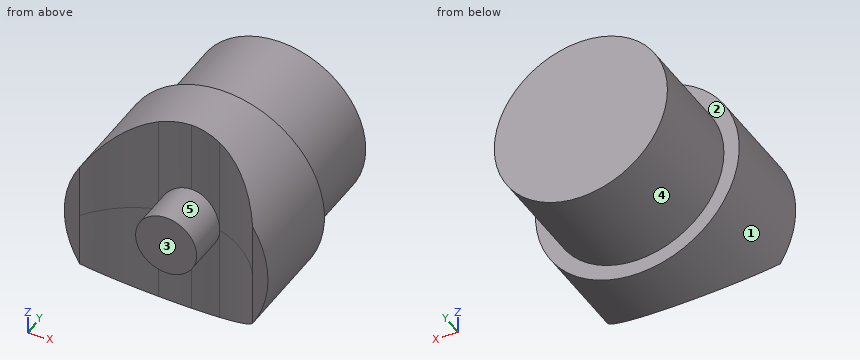
```python
from build123d import *

# Parameters (mm, degrees)
F0_W          = 1.5
F0_H          = 10
F0_W_2        = 8.5
F2_DEPTH      = 25
F2_DEPTH_BACK = 25


with BuildPart() as f1:
    # F0 (on Top) → F1 (revolve)
    with BuildSketch(Plane.XY):
        with BuildLine():
            Line((-10, 10), (-18.5, 10))
            Line((-18.5, 10), (-18.5, 0))
            ThreePointArc((-18.5, 0), (-16.099974277, 2.509062325), (-13, 4.0729282733))
            Line((-13, 4.0729282733), (-13, 4.5217803813))
            Line((-13, 4.5217803813), (-10, 4.5217803813))
            Line((-10, 4.5217803813), (-10, 10))
        make_face()
        with Locations((-19.25, 5)):
            Rectangle(F0_W, F0_H)
        with Locations((-14.25, 15)):
            Rectangle(F0_W_2, F0_H)
        with BuildLine():
            ThreePointArc((-13, 4.0729282733), (-11.516696098, 4.4089463041), (-10, 4.5217803813))
            Line((-10, 4.5217803813), (-13, 4.5217803813))
            Line((-13, 4.5217803813), (-13, 4.0729282733))
        make_face()
        with BuildLine():
            Line((-10, 0), (-10, 4.5217803813))
            ThreePointArc((-10, 4.5217803813), (-11.516696098, 4.4089463041), (-13, 4.0729282733))
            Line((-13, 4.0729282733), (-13, 0))
            Line((-13, 0), (-10, 0))
        make_face()
        with BuildLine():
            ThreePointArc((-13, 4.0729282733), (-16.099974277, 2.509062325), (-18.5, 0))
            Line((-18.5, 0), (-13, 0))
            Line((-13, 0), (-13, 4.0729282733))
        make_face()
    revolve(axis=Axis((-10, 10, 0), (0, -1, 0)))

    # F0 (on Top) → F2 (cut, two sides)
    with BuildSketch(Plane.XY) as f2_sk:
        with BuildLine():
            ThreePointArc((-13, 4.0729282733), (-16.099974277, 2.509062325), (-18.5, 0))
            Line((-18.5, 0), (-13, 0))
            Line((-13, 0), (-13, 4.0729282733))
        make_face()
        with BuildLine():
            Line((-7, 0), (-1.5, 0))
            ThreePointArc((-1.5, 0), (-3.900025723, 2.509062325), (-7, 4.0729282733))
            Line((-7, 4.0729282733), (-7, 0))
        make_face()
        with BuildLine():
            Line((-10, 0), (-10, 4.5217803813))
            ThreePointArc((-10, 4.5217803813), (-11.516696098, 4.4089463041), (-13, 4.0729282733))
            Line((-13, 4.0729282733), (-13, 0))
            Line((-13, 0), (-10, 0))
        make_face()
        with BuildLine():
            ThreePointArc((-7, 4.0729282733), (-8.483303902, 4.4089463041), (-10, 4.5217803813))
            Line((-10, 4.5217803813), (-10, 0))
            Line((-10, 0), (-7, 0))
            Line((-7, 0), (-7, 4.0729282733))
        make_face()
    extrude(amount=F2_DEPTH, mode=Mode.SUBTRACT)
    extrude(f2_sk.sketch, amount=-F2_DEPTH_BACK, mode=Mode.SUBTRACT)

    # F0 (on Top) → F3 (revolve)
    with BuildSketch(Plane.XY):
        with BuildLine():
            Line((-10, 0), (-10, 4.5217803813))
            ThreePointArc((-10, 4.5217803813), (-11.516696098, 4.4089463041), (-13, 4.0729282733))
            Line((-13, 4.0729282733), (-13, 0))
            Line((-13, 0), (-10, 0))
        make_face()
        with BuildLine():
            ThreePointArc((-13, 4.0729282733), (-11.516696098, 4.4089463041), (-10, 4.5217803813))
            Line((-10, 4.5217803813), (-13, 4.5217803813))
            Line((-13, 4.5217803813), (-13, 4.0729282733))
        make_face()
    revolve(axis=Axis((-10, 10, 0), (0, -1, 0)))


solid = f1.part
```
Can you work these out from the model? Positions are in its coordinate system, mm. Face numbers are marked on the shaded views. A direction names the side the tool comes from. Coordinates: 2 decimals unless noted, no trailing zeros. Order: outer loops, then holes, each group sorted by start corner. A loop starts at its lowest first (then second) coordinate and runs counter-clockwise, first axis right, second up.
1. If we section it at B-B (x = -3.5): Please give me the cut outline in (y, z).
2. Thinking about a two-plate mould opening in X: for the marked faces 3, 4 and 5, which applies, +X half, -X half, draft (parallel to the pull), parting line (faces both ways), or undercut?
3. For the marked faces 1 and 2, which set-ups out of +Z, -Z, +X, -X, +Y, -Y let a thin tool reach every point of the face, with its end or its side?
4. If we section it at D-D (z = 7): Please give me the cut outline in (x, y).
5. If we section it at C-C (y = 8.25): Please give me the cut outline in (x, z).
6. If we section it at A-A (y = 3.5): Please give me the cut outline in (x, z), then the cut area to 3 significant figures.
7. I'm going to push flat-ended pins straight in: pin 1 (2 mm diameter, centred on y = 14.5, z = -4, fed in from +X); pin 2 (3 mm diameter, centred on x = -4, y = 17, fed in from +Z); pin 3 (2 mm diameter, centred on x = -6.5, y = 17.5, fed in from +Z). Where does each tip first touch, or does it pass through?
8. I need wall thicknesses on line 1 (Y direction, x = -9.75, z = -8); line 2 (Y direction, x = -6, z = -0.25); line 3 (X direction, y = 6.5, z = 1.75). Which ranges of each line are inside material? Lowest first, please.
Entries:
1. outline: (2.2, -7.6) - (10, -7.6) - (10, -5.48) - (20, -5.48) - (20, 5.48) - (10, 5.48) - (10, 7.6) - (2.2, 7.6) - close
2. face 3: draft
2. face 4: parting line
2. face 5: undercut
3. face 1: +Y, -Y
3. face 2: +Y
4. outline: (-17.14, 1.62) arc R10.25 cw to (-2.86, 1.62) - (-2.86, 10) - (-5.18, 10) - (-5.18, 20) - (-14.82, 20) - (-14.82, 10) - (-17.14, 10) - close
5. outline: circle Ø20 at (-10, 0)
6. outline: (-14.46, -8.95) - (-14.46, 8.95) arc R10 ccw to start; circle Ø6 at (-10, 0); (-5.54, -8.95) arc R10 ccw to (-5.54, 8.95) - close
6. area: 170 mm2
7. pin 1: stops at x = -2.05
7. pin 2: stops at z = 7.21
7. pin 3: stops at z = 8.12
8. line 1: y = 4.52 to 20
8. line 2: y = 3.71 to 20
8. line 3: x = -19.85 to -0.15
